CAD build for the part. Positions are in the model's coordinates, mm. A direction names the side the tool comes from. Round coordinates to 2 decimals unless told otherwise and drop trailing zeros. Order: outer loops, then holes, each group sorted by start corner. A loop starts at its lowest first (then second) coordinate and runs counter-clockwise, first axis right, second up. Notation, with made-up numbers: M 76,-13.5 L 125,-13.5 A22 ccw 125,11.5 Z; hole C 69,80.5 d11. An arc over 180 degrees is marked long. Put each result on its own line as item: value.
```python
from build123d import *

# Parameters (mm, degrees)
CROQUIS1_R              = 1.5
CROQUIS1_R_2            = 4
SALIENTE_EXTRUIR1_DEPTH = 6
CROQUIS4_R              = 1.5
CORTAR_EXTRUIR3_DEPTH   = 54.749418602
CROQUIS5_R              = 1.5
CORTAR_EXTRUIR4_DEPTH   = 68.111846942
CROQUIS6_R              = 3.25
CORTAR_EXTRUIR5_DEPTH   = 5
CROQUIS7_R              = 3.25
CORTAR_EXTRUIR6_DEPTH   = 5


with BuildPart() as part:
    # Croquis1 → Saliente-Extruir1 (new body)
    with BuildSketch(Plane.XY):
        with BuildLine():
            Line((0, 0), (38, 0))
            ThreePointArc((38, 0), (40.828427125, -1.171572875), (42, -4))
            Line((42, -4), (42, -5))
            ThreePointArc((42, -5), (40.828427125, -7.828427125), (38, -9))
            Line((38, -9), (21, -9))
            ThreePointArc((21, -9), (12.514718626, -12.514718626), (9, -21))
            Line((9, -21), (9, -38))
            ThreePointArc((9, -38), (7.828427125, -40.828427125), (5, -42))
            Line((5, -42), (0, -42))
            ThreePointArc((0, -42), (-7.071067812, -39.071067812), (-10, -32))
            Line((-10, -32), (-10, 10))
            ThreePointArc((-10, 10), (-8.535533906, 13.535533906), (-5, 15))
            Line((-5, 15), (0, 15))
            Line((0, 15), (0, 0))
        make_face()
        with Locations((36, -5.58)):
            Circle(CROQUIS1_R, mode=Mode.SUBTRACT)
        with Locations((5, -5.58)):
            Circle(CROQUIS1_R, mode=Mode.SUBTRACT)
        with Locations((5, -36.58)):
            Circle(CROQUIS1_R, mode=Mode.SUBTRACT)
        with Locations((0, -21.1)):
            Circle(CROQUIS1_R_2, mode=Mode.SUBTRACT)
    extrude(amount=SALIENTE_EXTRUIR1_DEPTH)

    # Croquis4 → Cortar-Extruir3 (cut, through all)
    with BuildSketch(Plane.XZ.offset(9)):
        with Locations((25, 3)):
            Circle(CROQUIS4_R)
    extrude(amount=-CORTAR_EXTRUIR3_DEPTH, mode=Mode.SUBTRACT)

    # Croquis5 → Cortar-Extruir4 (cut, through all)
    with BuildSketch(Plane.ZY.offset(10)):
        with Locations((3, 5)):
            Circle(CROQUIS5_R)
    extrude(amount=-CORTAR_EXTRUIR4_DEPTH, mode=Mode.SUBTRACT)

    # Croquis6 → Cortar-Extruir5 (cut)
    with BuildSketch(Plane.XZ.offset(9)):
        with Locations((25, 3)):
            Circle(CROQUIS6_R)
    extrude(amount=-CORTAR_EXTRUIR5_DEPTH, mode=Mode.SUBTRACT)

    # Croquis7 → Cortar-Extruir6 (cut)
    with BuildSketch(Plane.ZY.offset(10)):
        with Locations((3, 5)):
            Circle(CROQUIS7_R)
    extrude(amount=-CORTAR_EXTRUIR6_DEPTH, mode=Mode.SUBTRACT)


solid = part.part
```
Item 1: Band-saw the part on C-C on y = -13.5. Give the cut face in (x, z), and give its area (3 significant figures).
Answers below:
outline: M -10,0 L 11.63,0 L 11.63,6 L -10,6 Z
area: 130 mm²
Item 2: Probe line 1 along Y through (x, z) = (5, 3); line 2 along Y through (x, z) = (-1, 4); line 3 along Z through (x, y) = (25, -1). List the from-to ranges inside material, lowest first. Write a range as [from, to].
Answers below:
line 1: [-42, -38.08], [-35.08, -7.08], [-4.08, 0]
line 2: [-41.95, -24.97], [-17.23, 3.88], [6.12, 15]
line 3: [0, 1.5], [4.5, 6]
Item 3: Mould opens along Y. For faces 4 (the flat face through (3, -42, 3)), 5 (the cylindrical face through (23.5, -2.03, 3.07)), 6 (the cylindrical face through (5.806, -4.315, 2.958)) say: pulls with the +Y half, pulls with the -Y half, needs draft (parallel to the pull), parting line crosses it, or undercut.
Answers below:
face 4: pulls with the -Y half
face 5: needs draft
face 6: undercut
Item 4: Pin check, flat tips, straight feed: P1, Ø3, axis at y = 9.5, z = 4, coming from the +X side; P2, Ø3, axis at x = 22, z = 4.5, coming from the -Y side; P3, Ø5, axis at x = 0, y = -21.1, coming from the -Z side; P4, Ø5, axis at x = 5, y = -5.58, coming from the -Z side. Stop position of each tip, or through.
Answers below:
P1: x = 0
P2: y = -9.01
P3: through
P4: z = 0
Item 5: Tool access for faces 1 (the flat face through (32, -9, 3)), 2 (the flat face through (0, 8, 3)), 3 (the cylindrical face through (-7.54, 1.75, 2.95)): list every direction of +Z, -Z, +X, -X, +Y, -Y with a clear straight run to the whole face (end or side of a thin tool).
Answers below:
face 1: +Z, -Z, +X, -Y
face 2: +Z, -Z, +X, +Y
face 3: -X
Item 6: Band-saw the part on A-A on x = 25. Give the cut face in (y, z).
Answers below:
outline: M -4,0 L 0,0 L 0,1.5 L -4,1.5 Z; M -4,4.5 L 0,4.5 L 0,6 L -4,6 Z
Item 7: Band-saw the part on B-B on y = 5. Give the cut face in (x, z), and give its area (3 significant figures).
Answers below:
outline: M -5,0 L 0,0 L 0,1.5 L -5,1.5 Z; M -5,4.5 L 0,4.5 L 0,6 L -5,6 Z
area: 15.0 mm²
Item 8: Band-saw the part on D-D on x = 12. Give the cut face in (y, z), and give its area (3 significant figures).
Answers below:
outline: M -13.06,0 L 0,0 L 0,6 L -13.06,6 Z
area: 78.4 mm²
